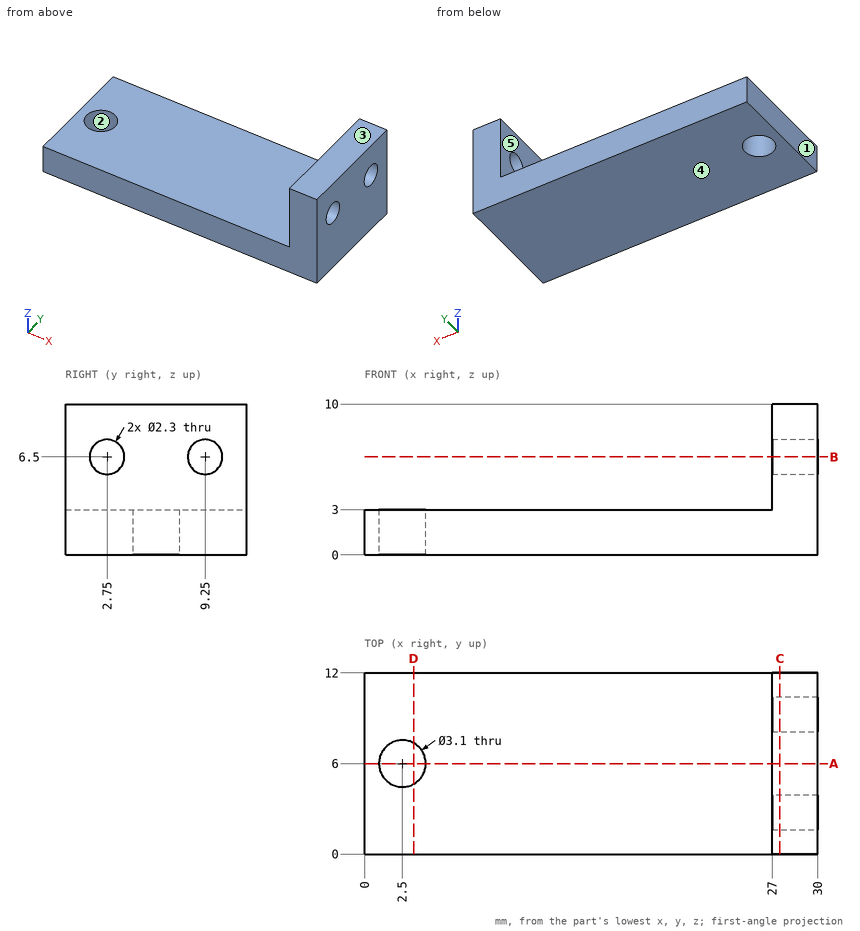
Print and shaded views of the part. All mm, measured from the part's lowest x, y and z. A direction names the side the tool comes from. Round coordinates to 2 decimals unless told otherwise and drop trailing zeros. Write each loop counter-clockwise with the first axis right and the second up, starting at its lowest first coordinate (ties: lowest second). Pieces come first, ordered by that corner, then holes. Notation, with made-up numbers: (57, 15.5) - (112, 15.5) arc R22 ccw to (112, 23.5) - close; hole circle Ø7 at (5.5, 12). An arc over 180 degrees is marked (long way). One line per item, written item: value.
(1) Cut at D-D, the plane x = 3.25. Give the cut face in (y, z), plus the area to 3 significant figures.
Values follow:
outline: (0, 0) - (4.64, 0) - (4.64, 3) - (0, 3) - close; (7.36, 0) - (12, 0) - (12, 3) - (7.36, 3) - close
area: 27.9 mm²
(2) Wall check: probe 1 along Y at (x, z) = (2.5, 0.9); probe 2 along Z at (x, y) = (28.25, 9.25); probe 3 along Z at (x, y) = (14, 4). Give the ranges that are in metal, low to high.
Values follow:
probe 1: y = 0 to 4.45, 7.55 to 12
probe 2: z = 0 to 5.35, 7.65 to 10
probe 3: z = 0 to 3
(3) Two-plate mould, pull along X, no slides. Class the marked faces 1, 2 and 3: pulls with the +X half, pulls with the -X half, needs draft (parallel to the pull), parting line crosses it, or undercut.
Values follow:
face 1: pulls with the -X half
face 2: undercut
face 3: needs draft
(4) Cut at C-C, the plane x = 27.5. Give the cut face in (y, z), plus the area to 3 significant figures.
Values follow:
outline: (0, 0) - (12, 0) - (12, 10) - (0, 10) - close; hole circle Ø2.3 at (2.75, 6.5); hole circle Ø2.3 at (9.25, 6.5)
area: 112 mm²
(5) Cut at A-A, the plane y = 6. Give the cut face in (x, z), plus the area to 3 significant figures.
Values follow:
outline: (0, 0) - (0.95, 0) - (0.95, 3) - (0, 3) - close; (4.05, 0) - (30, 0) - (30, 10) - (27, 10) - (27, 3) - (4.05, 3) - close
area: 102 mm²
(6) 3-axis set-ups, long thin cutter, end or side, ignore diameter. For the marked faces 4 and 5: which of +Z, -Z, +X, -X, +Y, -Y reach the whole face in a straight line?
Values follow:
face 4: -Z, +X, -X, +Y, -Y
face 5: +Z, -X, +Y, -Y
(7) Drop flat-ended pins along their axis: P1, Ø5, axis at x = 7, y = 7.5, coming from the +Z side; P2, Ø5.5, axis at y = 5, z = 6.5, coming from the -X side; P3, Ø1.9, axis at x = 2.5, y = 6, coming from the +Z side. Give the stop position or say it passes through.
Values follow:
P1: stops at z = 3
P2: stops at x = 27
P3: passes through
(8) Cut at B-B, the plane z = 6.5. Give the cut face in (x, y).
Values follow:
outline: (27, 0) - (30, 0) - (30, 1.6) - (27, 1.6) - close; (27, 3.9) - (30, 3.9) - (30, 8.1) - (27, 8.1) - close; (27, 10.4) - (30, 10.4) - (30, 12) - (27, 12) - close
